Read the model definition and answer for the solid it produces. Units are mm, in the model's axes. Face numbers are marked on the shaded views. A direction names the side the tool comes from. Give positions to 0.01 mm unless a question says otherwise; leave off trailing zeros. Write each loop counter-clockwise with the first axis right and the second up, starting at its lowest first coordinate (ties: lowest second). Pieces come first, ordered by that corner, then holes. Notation, with made-up numbers: (-3.5, 77.25) - (47.5, 77.25) arc R9 cw to (47.5, 91.25) - close; hole circle Ø8 at (50.25, 5.25). An arc over 180 degrees is marked (long way). Use CSV: the item, a comma, the result in double quotes. Start each with the question number.
from build123d import *

# Parameters (mm, degrees)
F1_DEPTH = 85
F0_W     = 13.8709768653
F0_H     = 16.2702709436
F0_W_2   = 16.0746378824
F0_H_2   = 12.2704952955
F2_DEPTH = 25
F3_DEPTH = 93
F4_DEPTH = 25


with BuildPart() as f1:
    # F0 (on Front) → F1 (new body)
    with BuildSketch(Plane.XZ):
        Polygon((-61.2078905106, -141.2702709436), (-75.0788673759, -141.2702709436), (-123.6273050308, -141.2702709436), (-123.6273050308, -291.2702709436), (16.3726949692, -291.2702709436), (16.3726949692, -199.5083987713), (16.3726949692, -187.2379034758), (16.3726949692, -141.2702709436), align=None)
    extrude(amount=F1_DEPTH)

    # F0 (on Front) → F2 (join)
    with BuildSketch(Plane.XZ):
        with Locations((-68.1433789432, -133.1351354718)):
            Rectangle(F0_W, F0_H)
        with Locations((24.4100139104, -193.3731511235)):
            Rectangle(F0_W_2, F0_H_2)
    extrude(amount=F2_DEPTH)

    # F0 (on Front) → F3 (join)
    with BuildSketch(Plane.XZ):
        Polygon((125, 125), (-125, 125), (-125, -125), (-75.0788673759, -125), (-61.2078905106, -125), (125, -125), align=None)
    extrude(amount=F3_DEPTH)

    # F0 (on Front) → F4 (join)
    with BuildSketch(Plane.XZ):
        Polygon((32.4473328516, -141.2702709436), (32.4473328516, -187.2379034758), (32.4473328516, -199.5083987713), (32.4473328516, -221.2702709436), (142.4473328516, -221.2702709436), (142.4473328516, -141.2702709436), align=None)
    extrude(amount=F4_DEPTH)


solid = f1.part
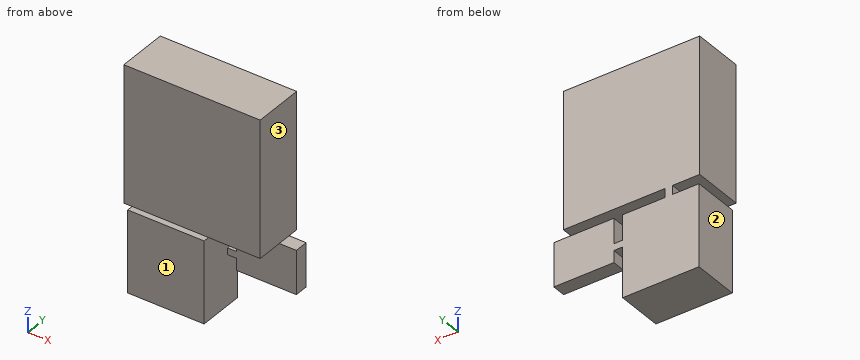
(1) The part is cut by section B-B on x = 97. Write down the section's boundary in (y, z), plus the area to 4 significant figures.
(2) The part is cut by section D-D on z = -2.5. Write down the section's boundary in (x, y), plus the area to 4 significant figures.
(3) The part is cut by section A-A on y = -52. Write down the section's boundary in (x, z), plus the area to 3 significant figures.
(4) Consider probe 1 along Z at (x, y) = (105, -11.5); probe 2 along Z at (x, y) = (-96, -36); probe 3 along X at (y, z) = (-24, -148.5). Determine where each line is inside the solid, lowest interval first.
(5) Given P1, Ø11, axis at y = -8, z = -207.5, coming from the -X side; P2, Ø1, axis at x = -91, z = -203.5, coming from the -Y side; P3, Ø8, axis at y = -17.5, z = -133, coming from the +X side, each flat-ended and moving along its own axis, determine where each tip first touches the part or whether it passes through.
(6) The part is cut by section C-C on y = -9. Write down the section's boundary in (x, z).
(7) Which of the six approach directions +Z, -Z, +X, -X, +Y, -Y give full straight-line access (tool end or side, diameter ignored) to the marked faces 1, 2 and 3?
Reported:
1,outline,"(-93, -125) - (0, -125) - (0, 125) - (-93, 125) - close; (-25, -221.27) - (0, -221.27) - (0, -141.27) - (-25, -141.27) - close"
1,area,"25,250 mm²"
2,outline,"(-125, -93) - (125, -93) - (125, 0) - (-125, 0) - close"
2,area,"23,250 mm²"
3,outline,"(-125, -125) - (125, -125) - (125, 125) - (-125, 125) - close; (-123.63, -291.27) - (16.37, -291.27) - (16.37, -141.27) - (-123.63, -141.27) - close"
3,area,"83,500 mm²"
4,probe 1,"-221.27 to -141.27, -125 to 125"
4,probe 2,"-291.27 to -141.27, -125 to 125"
4,probe 3,"-123.63 to 16.37, 32.45 to 142.45"
5,P1,"x = -123.63"
5,P2,"y = -85"
5,P3,"x = -61.21"
6,outline,"(-125, -125) - (-75.08, -125) - (-75.08, -141.27) - (-123.63, -141.27) - (-123.63, -291.27) - (16.37, -291.27) - (16.37, -199.51) - (32.45, -199.51) - (32.45, -221.27) - (142.45, -221.27) - (142.45, -141.27) - (32.45, -141.27) - (32.45, -187.24) - (16.37, -187.24) - (16.37, -141.27) - (-61.21, -141.27) - (-61.21, -125) - (125, -125) - (125, 125) - (-125, 125) - close"
7,face 1,"-Z, +X, -X, -Y"
7,face 2,"-Z, -X, +Y, -Y"
7,face 3,"+Z, +X, +Y, -Y"
